from build123d import *

# Parameters (mm, degrees)
BOSS_EXTRUDE1_DEPTH = 425


with BuildPart() as part:
    # Sketch1 → Boss-Extrude1 (new body)
    with BuildSketch(Plane.XY.offset(425)):
        with BuildLine():
            Line((-20, 0.5), (-19.5, 0))
            Line((-19.5, 0), (-6, 0))
            Line((-6, 0), (-5.8, 0.2))
            Line((-5.8, 0.2), (5.8, 0.2))
            Line((5.8, 0.2), (6, 0))
            Line((6, 0), (19.5, 0))
            Line((19.5, 0), (20, 0.5))
            Line((20, 0.5), (20, 3.708496771))
            ThreePointArc((20, 3.708496771), (20.081946856, 3.914537598), (20.283018838, 4.008015763))
            ThreePointArc((20.283018838, 4.008015763), (22.487270957, 13.337451356), (15.548604796, 6.722921305))
            ThreePointArc((15.548604796, 6.722921305), (15.569235136, 6.501321924), (15.431520983, 6.326488551))
            Line((15.431520983, 6.326488551), (13.999999829, 5.499999462))
            Line((13.999999829, 5.499999462), (0.499999829, 5.499999462))
            Line((0.499999829, 5.499999462), (-1.71e-07, 5.211324462))
            Line((-1.71e-07, 5.211324462), (-0.500000171, 5.499999462))
            Line((-0.500000171, 5.499999462), (-14.000000171, 5.499999462))
            Line((-14.000000171, 5.499999462), (-15.431521324, 6.326488551))
            ThreePointArc((-15.431521324, 6.326488551), (-15.569235521, 6.501321979), (-15.548605174, 6.72292143))
            ThreePointArc((-15.548605174, 6.72292143), (-22.487271055, 13.33745115), (-20.283018868, 4.008016016))
            ThreePointArc((-20.283018868, 4.008016016), (-20.081946865, 3.914537846), (-20, 3.708497))
            Line((-20, 3.708497), (-20, 0.5))
        make_face()
    extrude(amount=-BOSS_EXTRUDE1_DEPTH)


solid = part.part
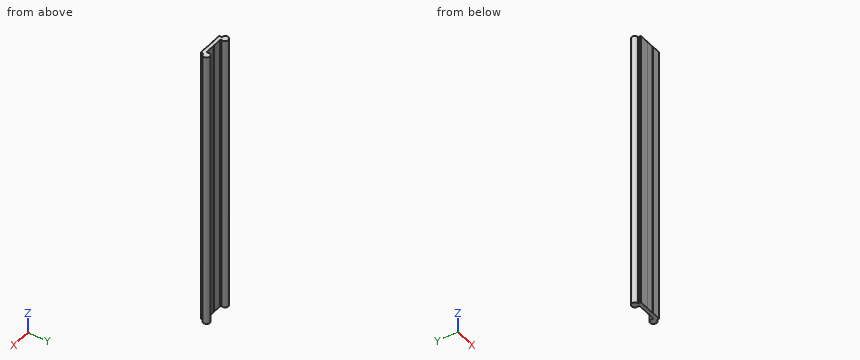
Input: part model. Units: mm. Frame: model coordinates. Coordinates: 2 decimals unless noted, no trailing zeros. Loops run counter-clockwise (first coordinate to the right, second up) from the corner with the lowest first, then second, coordinate; pieces in that order, holes last.
(1) First-contact query: pin 1 Ø3.5 at (y, z) = (2, 122) entering from -X; pin 2 Ø11 at (x, z) = (5.5, 262) entering from +Y; pin 3 Ø3 at (y, z) = (11, 73) entering from -X; pin 4 Ø1.5 at (x, y) = (-4.5, 7) entering from -Z. Flat tips, straight axial feed; report the tip coordinate or a pass-through.
(2) Material intervals for probe 1 along Y at (x, z) = (5, 322); probe 2 along Y at (x, z) = (10.5, 23.5); probe 3 along X at (y, z) = (11.5, 41), sorted ascending.
(3) Section A-A on y = 9. Return the cut outline in (x, z), then the cut area to 3 significant figures.
(4) Section B-B on z = 363. Return the cut outline in (x, y).
Data:
1. pin 1: stops at x = -20
1. pin 2: stops at y = 5.5
1. pin 3: stops at x = -24.97
1. pin 4: passes through
2. probe 1: y = 0.2 to 5.5
2. probe 2: y = 0 to 5.5
2. probe 3: x = -24.33 to -15.67, 15.67 to 24.33
3. outline: (-25, 0) - (-15, 0) - (-15, 425) - (-25, 425) - close; (15, 0) - (25, 0) - (25, 425) - (15, 425) - close
3. area: 8,500 mm2
4. outline: (-20.28, 4.01) arc R0.3 cw to (-20, 3.71) - (-20, 0.5) - (-19.5, 0) - (-6, 0) - (-5.8, 0.2) - (5.8, 0.2) - (6, 0) - (19.5, 0) - (20, 0.5) - (20, 3.71) arc R0.3 cw to (20.28, 4.01) arc R5 ccw (long way) to (15.55, 6.72) arc R0.3 cw to (15.43, 6.33) - (14, 5.5) - (0.5, 5.5) - (0, 5.21) - (-0.5, 5.5) - (-14, 5.5) - (-15.43, 6.33) arc R0.3 cw to (-15.55, 6.72) arc R5 ccw (long way) to start
